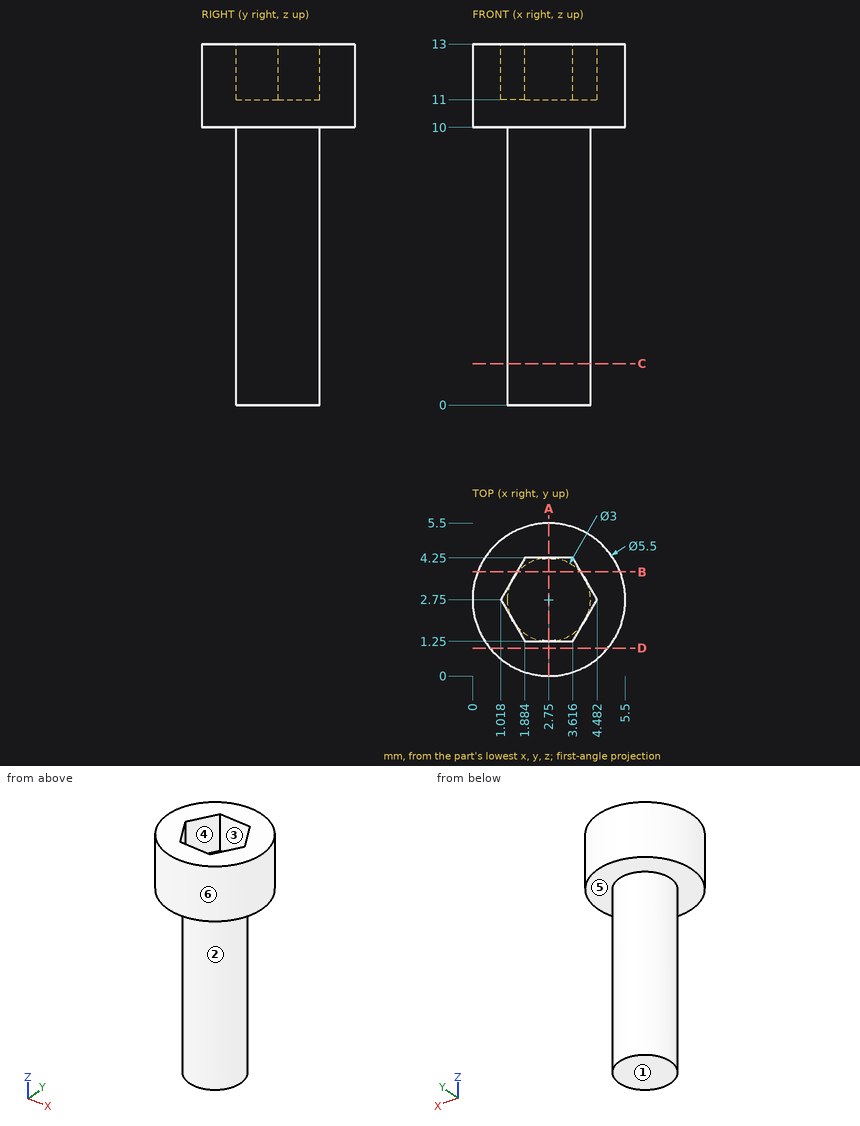
For this review, use the dimensioned drawing (mm, ordinates from the lowest corner) and the shaded views. A direction names the side the tool comes from. Round coordinates to 2 decimals unless told otherwise and drop trailing zeros. Write each loop counter-clockwise with the first axis right and the second up, starting at its lowest first coordinate (ties: lowest second). Pieces come first, ordered by that corner, then holes. Notation, with made-up numbers: M -29.5,-3.5 L 4.5,-3.5 A14 ccw 4.5,0.5 Z; hole C -31,-35 d11. An arc over 180 degrees is marked long. Write item = value, one per line. Start each with the question number.
(1) Clearance check with flat-ended pins moving along their axes: pin 1 Ø2.5 at (x, y) = (3.5, 2.5) entering from +Z; pin 2 Ø2 at (x, z) = (3, 6.5) entering from +Y. State where each tip first meets the part, or that it passes through.
(2) We need section B-B (y = 3.75). Give the boundary of the cut face in (x, z), then the cut area to 3 significant figures.
(3) For the marked faces 1 and 2, list the 3-axis set-ups (+Z, -Z, +X, -X, +Y, -Y) from which the entire face can be reached by the end or side of a thin tool; tool diameter is ignored.
(4) We need section A-A (x = 2.75). Give the boundary of the cut face in (y, z), then the cut area to 3 significant figures.
(5) The part is to be moulded in two halves that separate along Y. For the marked faces 3, 4, 5 and 6, say which applies: +Y half, -Y half, draft (parallel to the pull), parting line (faces both ways), or undercut.
(6) We need section D-D (y = 1). Give the boundary of the cut face in (x, z).
(7) For line 1 along Z through (x, y) = (3.4, 0.9); line 2 along Z through (x, y) = (3, 2.6); line 3 along X through (y, z) = (2.7, 12.25), list the stretches that pass through material, from the lowest coordinate up.
(8) We need section C-C (z = 1.5). Give the boundary of the cut face in (x, y), then the cut area to 3 significant figures.
Results found:
q1.pin_1 = 13
q1.pin_2 = 4.25
q2.outline = M 0.19,10 L 1.63,10 L 1.63,0 L 3.87,0 L 3.87,10 L 5.31,10 L 5.31,13 L 3.9,13 L 3.9,11 L 1.6,11 L 1.6,13 L 0.19,13 Z
q2.area = 33.1 mm²
q3.face_1 = -Z, +X, -X, +Y, -Y
q3.face_2 = -Z
q4.outline = M 0,10 L 1.25,10 L 1.25,0 L 4.25,0 L 4.25,10 L 5.5,10 L 5.5,13 L 4.25,13 L 4.25,11 L 1.25,11 L 1.25,13 L 0,13 Z
q4.area = 40.5 mm²
q5.face_3 = undercut
q5.face_4 = undercut
q5.face_5 = draft
q5.face_6 = parting line
q6.outline = M 0.63,10 L 4.87,10 L 4.87,13 L 0.63,13 Z
q7.line_1 = 10 to 13
q7.line_2 = 0 to 11
q7.line_3 = 0 to 1.05, 4.45 to 5.5
q8.outline = C 2.75,2.75 d3
q8.area = 7.07 mm²
